Could you check a few things on this model? Use its own coordinates, in mm. A direction names the side the tool comes from. Coordinates: 2 decimals unless noted, no trailing zeros. Write each loop counter-clockwise with the first axis right and the second up, starting at its lowest first coordinate (ties: lowest second). Pieces come first, ordered by that corner, then holes. Notation, with made-up numbers: (60.5, -1.75) - (104.5, -1.75) arc R30 cw to (104.5, 35.25) - close; hole circle Ø2 at (3.25, 3.25). An arc over 180 degrees is marked (long way). Answer as a JSON object with one key per item and string values. Group by question number.
1) If we section it at B-B (x = 4): Write out the boundary of the cut face in (y, z).
2) If we section it at D-D (x = -6): Write out the boundary of the cut face in (y, z), plus the area to 3 significant figures.
3) If we section it at C-C (z = 2.25): Write out the boundary of the cut face in (x, y).
4) Please list where these lines run through material, in increasing order: line 1 along Y through (x, z) = (-6, 11.25); line 2 along Y through (x, z) = (4, 2.25); line 3 along Z through (x, y) = (-5.5, -13.25).
5) If we section it at A-A (y = 0): Write out the boundary of the cut face in (x, z), plus the area to 3 significant figures.
6) We'd pull the mould along Y, two halves only. Please class faces 1 (the flat face through (-6, -3.5, 13)), 2 (the cylindrical face through (-1.715, -3.801, 4.056)), 3 (the cylindrical face through (-6.1, -13.4, 15)): released by +Y, released by -Y, zero draft, split by the parting line, or undercut.
7) On a 3-axis mill with a long thin cutter (end or side, diameter ignored), from which of +Z, -Z, +X, -X, +Y, -Y can I reach the whole of each face in a straight line? I mean faces 4 (the flat face through (-14, -6.5, 2)), 5 (the cylindrical face through (-2.285, -3.801, 13.07)), 6 (the flat face through (-6, -7, 8)), 7 (the flat face through (-6, -18, 18)), 8 (the flat face through (-2, -12, 9)). Say none if no direction works.
8) Will these pins go through, and if not, where does the flat tip stop? pin 1 Ø0.8 at (x, y) = (-5.5, -21) entering from +Z; pin 2 Ø8 at (y, z) = (-6, 11) entering from -X; pin 3 Ø8 at (y, z) = (-16.5, 8) entering from +X; pin 4 Ø2.5 at (x, y) = (-4, 0) entering from -Z.
```python
from build123d import *

# Parameters (mm, degrees)
SKETCH_W        = 15
SKETCH_H        = 7
SKETCH_R        = 1.65
PAD_DEPTH       = 8
SKETCH001_W     = 8
SKETCH001_H     = 8
PAD001_DEPTH    = 20
PAD002_DEPTH    = 8
SKETCH003_R     = 1.4
POCKET_DEPTH    = 10
CHAMFER_SIZE    = 0.5
FILLET_R        = 3
FILLET001_R     = 1
FILLET002_R     = 1
FILLET003_R     = 1
SKETCH007_W     = 12
SKETCH007_H     = 3
PAD004_DEPTH    = 10
CHAMFER001_SIZE = 5
FILLET005_R     = 4
FILLET006_R     = 1.5


with BuildPart() as part:
    # Sketch (on XY_Plane of Origin) → Pad (new body)
    with BuildSketch(Plane.XY):
        Rectangle(SKETCH_W, SKETCH_H)
        with Locations((-4, 0)):
            Circle(SKETCH_R, mode=Mode.SUBTRACT)
        with Locations((4, 0)):
            Circle(SKETCH_R, mode=Mode.SUBTRACT)
    extrude(amount=PAD_DEPTH)

    # Sketch001 (on Face2 of Pad) → Pad001 (join)
    with BuildSketch(Plane.XZ.offset(3.5)):
        with Locations((-6, 4)):
            Rectangle(SKETCH001_W, SKETCH001_H)
    extrude(amount=PAD001_DEPTH)

    # Sketch002 (on Face5 of Pad001) → Pad002 (join)
    with BuildSketch(Plane(origin=(-10, 0, 0), x_dir=(0, -1, 0), z_dir=(-1, 0, 0))):
        with BuildLine():
            Line((3.5, 8), (23.5, 8))
            Line((23.5, 8), (23.5, 18))
            Line((23.5, 18), (17.372983, 18))
            ThreePointArc((9.627017, 18), (13.5, 15), (17.372983, 18))
            Line((3.5, 18), (9.627017, 18))
            Line((3.5, 8), (3.5, 18))
        make_face()
    extrude(amount=-PAD002_DEPTH)

    # Sketch003 (on Face3 of Pad002) → Pocket (cut)
    with BuildSketch(Plane.XY.offset(18)):
        with Locations((-6, -6.57)):
            Circle(SKETCH003_R)
        with Locations((-6, -20.43)):
            Circle(SKETCH003_R)
    extrude(amount=-POCKET_DEPTH, mode=Mode.SUBTRACT)

    # Chamfer
    chamfer_edges = [part.edges().sort_by_distance(p)[0] for p in [
        (-7.4, -20.43, 18),
        (-7.4, -6.57, 18),
    ]]
    chamfer(chamfer_edges, length=CHAMFER_SIZE)

    # Fillet
    fillet_edges = [part.edges().sort_by_distance(p)[0] for p in [
        (-7.5, 3.5, 4),
        (7.5, 3.5, 4),
        (7.5, -3.5, 4),
        (-2, -23.5, 9),
        (-10, -23.5, 9),
    ]]
    fillet(fillet_edges, radius=FILLET_R)

    # Fillet001
    fillet001_edges = [part.edges().sort_by_distance(p)[0] for p in [
        (-7.5, -3.5, 4),
        (-10, -3.5, 9),
    ]]
    fillet(fillet001_edges, radius=FILLET001_R)

    # Fillet002
    fillet002_edges = [part.edges().sort_by_distance(p)[0] for p in [
        (-2, -3.5, 4),
    ]]
    fillet(fillet002_edges, radius=FILLET002_R)

    # Fillet003
    fillet003_edges = [part.edges().sort_by_distance(p)[0] for p in [
        (-2, -3.5, 13),
    ]]
    fillet(fillet003_edges, radius=FILLET003_R)

    # Sketch007 (on Face11 of Fillet003) → Pad004 (join)
    with BuildSketch(Plane(origin=(-10, 0, 0), x_dir=(0, -1, 0), z_dir=(-1, 0, 0))):
        with Locations((12.5, 1.5)):
            Rectangle(SKETCH007_W, SKETCH007_H)
    extrude(amount=PAD004_DEPTH)

    # Chamfer001
    chamfer001_edges = [part.edges().sort_by_distance(p)[0] for p in [
        (-10, -12.5, 3),
    ]]
    chamfer(chamfer001_edges, length=CHAMFER001_SIZE)

    # Fillet005
    fillet005_edges = [part.edges().sort_by_distance(p)[0] for p in [
        (-15, -12.5, 3),
    ]]
    fillet(fillet005_edges, radius=FILLET005_R)

    # Fillet006
    fillet006_edges = [part.edges().sort_by_distance(p)[0] for p in [
        (-20, -6.5, 1.5),
        (-10, -6.5, 1.5),
        (-10, -18.5, 1.5),
        (-10, -18.5, 5.5),
        (-20, -18.5, 1.5),
        (-10, -6.5, 5.5),
    ]]
    fillet(fillet006_edges, radius=FILLET006_R)


solid = part.part
```
Here are the results:
{
 "1": {"outline": "(-3.5, 0) - (-1.65, 0) - (-1.65, 8) - (-3.5, 8) - close; (1.65, 0) - (3.5, 0) - (3.5, 8) - (1.65, 8) - close"},
 "2": {"outline": "(-23.5, 0) - (3.1, 0) - (3.1, 8) - (-3.5, 8) - (-3.5, 18) - (-4.67, 18) - (-5.17, 17.5) - (-5.17, 8) - (-7.97, 8) - (-7.97, 17.5) - (-8.47, 18) - (-9.63, 18) arc R4 cw to (-17.37, 18) - (-18.53, 18) - (-19.03, 17.5) - (-19.03, 8) - (-21.83, 8) - (-21.83, 17.5) - (-22.33, 18) - (-23.5, 18) - close", "area": "339 mm²"},
 "3": {"outline": "(-20, -17) arc R1.5 ccw to (-18.5, -18.5) - (-11.5, -18.5) arc R1.5 cw to (-10, -20) - (-10, -20.5) arc R3 ccw to (-7, -23.5) - (-5, -23.5) arc R3 ccw to (-2, -20.5) - (-2, -4.5) arc R1 cw to (-1, -3.5) - (4.5, -3.5) arc R3 ccw to (7.5, -0.5) - (7.5, 0.5) arc R3 ccw to (4.5, 3.5) - (-4.5, 3.5) arc R3 ccw to (-7.5, 0.5) - (-7.5, -2.5) arc R1 cw to (-8.5, -3.5) - (-9, -3.5) arc R1 ccw to (-10, -4.5) - (-10, -5) arc R1.5 cw to (-11.5, -6.5) - (-18.5, -6.5) arc R1.5 ccw to (-20, -8) - close; hole circle Ø3.3 at (-4, 0); hole circle Ø3.3 at (4, 0)"},
 "4": {"line 1": "y = -23.5 to -21.83, -19.03 to -7.97, -5.17 to -3.5", "line 2": "y = -3.5 to -1.65, 1.65 to 3.5", "line 3": "z = 0 to 15.01"},
 "5": {"outline": "(-7.5, 0) - (-5.65, 0) - (-5.65, 8) - (-7.5, 8) - close; (-2.35, 0) - (2.35, 0) - (2.35, 8) - (-2.35, 8) - close; (5.65, 0) - (7.5, 0) - (7.5, 8) - (5.65, 8) - close", "area": "67.2 mm²"},
 "6": {"face 1": "released by +Y", "face 2": "released by -Y", "face 3": "undercut"},
 "7": {"face 4": "+Z, -Z, -X, +Y", "face 5": "+Z, +X, +Y", "face 6": "+Z", "face 7": "+Z, +X, -X, +Y, -Y", "face 8": "+Z, -Z, +X, -Y"},
 "8": {"pin 1": "stops at z = 8", "pin 2": "stops at x = -10.98", "pin 3": "stops at x = -2", "pin 4": "passes through"}
}
